```python
from build123d import *

# Parameters (mm, degrees)
BOSS_EXTRUDE1_DEPTH = 10
SKETCH3_W           = 4.25
SKETCH3_H           = 6
CUT_EXTRUDE1_DEPTH  = 10
SKETCH4_R           = 1.5
CUT_EXTRUDE2_DEPTH  = 11


with BuildPart() as part:
    # Sketch2 → Boss-Extrude1 (new body)
    with BuildSketch(Plane(origin=(0, 0, 0), x_dir=(1, 0, 0), z_dir=(0, 1, 0))):
        with BuildLine():
            Line((0, -4.25), (29.5, -4.25))
            ThreePointArc((29.5, -4.25), (33.75, 0), (29.5, 4.25))
            Line((29.5, 4.25), (0, 4.25))
            ThreePointArc((0, 4.25), (-4.25, 0), (0, -4.25))
        make_face()
    extrude(amount=BOSS_EXTRUDE1_DEPTH)

    # Sketch3 → Cut-Extrude1 (cut)
    with BuildSketch(Plane.XY.offset(4.25)):
        Polygon((24.75, 10), (4.75, 10), (14.75, 4), align=None)
        Polygon((4.75, 6), (0, 6), (0, 0), (14.75, 0), align=None)
        with Locations((-2.125, 3)):
            Rectangle(SKETCH3_W, SKETCH3_H)
        Polygon((29.5, 0), (29.5, 6), (24.75, 6), (14.75, 0), align=None)
        with Locations((31.625, 3)):
            Rectangle(SKETCH3_W, SKETCH3_H)
    extrude(amount=-CUT_EXTRUDE1_DEPTH, mode=Mode.SUBTRACT)

    # Sketch4 → Cut-Extrude2 (cut, through all)
    with BuildSketch(Plane(origin=(0, 10, 0), x_dir=(1, 0, 0), z_dir=(0, 1, 0))):
        Circle(SKETCH4_R)
        with Locations((29.5, 0)):
            Circle(SKETCH4_R)
    extrude(amount=-CUT_EXTRUDE2_DEPTH, mode=Mode.SUBTRACT)


solid = part.part
```
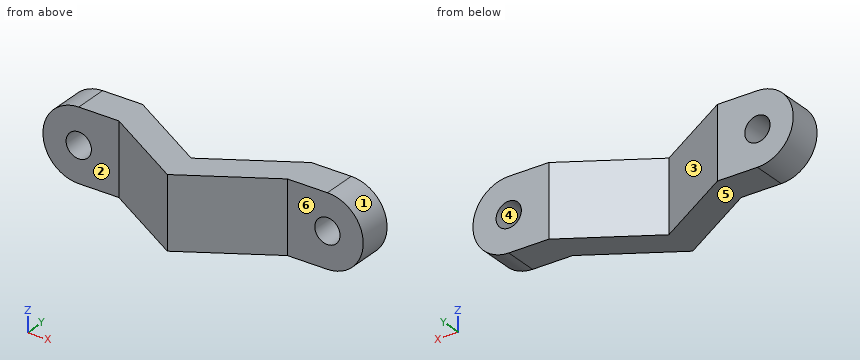
Work out the finished part from the listing and answer in its coordinate system (mm). Face numbers are marked on the shaded views. A direction names the side the tool comes from. Give positions to 0.01 mm unless a question says otherwise; leave off trailing zeros. Loops run counter-clockwise (first coordinate to the right, second up) from the corner with the lowest first, then second, coordinate; pieces in that order, holes last. Notation, with made-up numbers: (62, -17.5) -> (115, -17.5) arc R13 cw to (115, 6.5) -> close; hole circle Ø3 at (-32, -26.75). An arc over 180 degrees is marked (long way). Write item = value, one per line. Start each with the question number.
(1) Find section B-B on y = 8. Give the vertices of the cut face in (x, z), and give its area (3 significant figures).
(2) Find section C-C on y = 4.5. Give the vertices of the cut face in (x, z).
(3) The mould has two halves that part along Z. Classify the marked faces 4, 5 and 6: +Z half, -Z half, draft (parallel to the pull), parting line (faces both ways), or undercut.
(4) Find section D-D on z = -2. Give the vertices of the cut face in (x, y).
(5) Find section A-A on z = 0. Give the vertices of the cut face in (x, y).
(6) Given pin 1 Ø1 at (x, z) = (3, -2) entering from -Y; pin 2 Ø6 at (x, y) = (2.5, 4) entering from -Z; pin 3 Ø1.8 at (x, z) = (0, 0) entering from -Y; pin 4 Ø2 at (y, z) = (2.5, -1) entering from -X, each flat-ended and moving along its own axis, determine where each tip first touches the part or whether it passes through.
(7) Which of the six approach directions +Z, -Z, +X, -X, +Y, -Y give full straight-line access (tool end or side, diameter ignored) to the marked faces 1, 2 and 3?
(8) Find the intervals of material crossed by probe 1 along X at (y, z) = (7.8, 0); probe 2 along X at (y, z) = (7.7, 0); probe 3 along Z at (x, y) = (29.5, 7.2), in increasing order. Write a range as from..to.
From the geometry:
q1.outline = (0, -4.25) -> (8.08, -4.25) -> (8.08, 4.25) -> (0, 4.25) arc R4.25 ccw to start; (21.42, -4.25) -> (29.5, -4.25) arc R4.25 ccw to (29.5, 4.25) -> (21.42, 4.25) -> close; hole circle Ø3 at (0, 0); hole circle Ø3 at (29.5, 0)
q1.area = 180 mm^2
q2.outline = (7.25, -4.25) -> (13.92, -4.25) -> (13.92, 4.25) -> (7.25, 4.25) -> close; (15.58, -4.25) -> (22.25, -4.25) -> (22.25, 4.25) -> (15.58, 4.25) -> close
q3.face_4 = undercut
q3.face_5 = -Z half
q3.face_6 = draft
q4.outline = (-3.75, 6) -> (4.75, 6) -> (14.75, 0) -> (24.75, 6) -> (33.25, 6) -> (33.25, 10) -> (24.75, 10) -> (14.75, 4) -> (4.75, 10) -> (-3.75, 10) -> close
q5.outline = (-4.25, 6) -> (-1.5, 6) -> (-1.5, 10) -> (-4.25, 10) -> close; (1.5, 6) -> (4.75, 6) -> (14.75, 0) -> (24.75, 6) -> (28, 6) -> (28, 10) -> (24.75, 10) -> (14.75, 4) -> (4.75, 10) -> (1.5, 10) -> close; (31, 6) -> (33.75, 6) -> (33.75, 10) -> (31, 10) -> close
q6.pin_1 = 6
q6.pin_2 = -4.25
q6.pin_3 = through
q6.pin_4 = 8.92
q7.face_1 = +X, +Y, -Y
q7.face_2 = +Z, -Z, -X, -Y
q7.face_3 = +Z, -Z, +Y
q8.probe_1 = -4.25..-1.5, 1.5..8.42, 21.08..28, 31..33.75
q8.probe_2 = -4.25..-1.5, 1.5..8.58, 20.92..28, 31..33.75
q8.probe_3 = -4.25..-1.5, 1.5..4.25
